The model under review builds one solid part; all positions refer to its coordinate system, in mm. Give positions to 0.01 mm unless a question says otherwise; leave off trailing zeros. Loops run counter-clockwise (first coordinate to the right, second up) from the corner with the lowest first, then second, coordinate; pieces in that order, holes last. Notation, with made-up numbers: M 60.25,-35 L 79.25,-35 A29 cw 79.25,-11 Z; hole C 76,-14.5 d1. An arc over 180 degrees is marked long. Write item = value, one per line. Start each with the question number.
1. We need section A-A on z = 5. Give the boundary of the cut face in (x, y), then the cut area to 3 significant figures.
2. We need section B-B on y = 1.4. Give the boundary of the cut face in (x, z) (3 decimals).
3. Wall thickness on line 1 along Z through (x, y) = (5, 2.8) (3 decimals); line 2 along X through (y, z) = (0.95, -5); line 3 along X through (y, z) = (0.7, -1): over which ranges is each line inside the solid? List them lowest first. Write a range as from..to.
4. We need section C-C on x = 6. Give the boundary of the cut face in (y, z) (3 decimals).
from build123d import *

# Parameters (mm, degrees)
F0_W     = 38.1
F0_H     = 19.05
F0_W_2   = 25.4
F0_H_2   = 1.27
F1_DEPTH = 4.7498
F2_R     = 3.175
F3_R     = 0.7874


with BuildPart() as f1:
    # F0 (on Front) → F1 (new body)
    with BuildSketch(Plane.XZ):
        Rectangle(F0_W, F0_H)
        with Locations((0, -4.7498)):
            Rectangle(F0_W_2, F0_H_2, mode=Mode.SUBTRACT)
        with Locations((0, 4.7498)):
            Rectangle(F0_W_2, F0_H_2, mode=Mode.SUBTRACT)
    extrude(amount=-F1_DEPTH)

    # F2
    f2_edges = [f1.edges().sort_by_distance(p)[0] for p in [
        (19.05, 2.3749, 9.525),
        (19.05, 2.3749, -9.525),
        (-19.05, 2.3749, 9.525),
        (-19.05, 2.3749, -9.525),
    ]]
    fillet(f2_edges, radius=F2_R)

    # F3
    f3_edges = [f1.edges().sort_by_distance(p)[0] for p in [
        (19.05, 0, 0),
        (18.120064, 0, -8.595064),
        (18.120064, 0, 8.595064),
        (0, 0, -9.525),
        (0, 0, 9.525),
        (-18.120064, 0, -8.595064),
        (-18.120064, 0, 8.595064),
        (-19.05, 0, 0),
        (-12.7, 0, -4.7498),
        (0, 0, -4.1148),
        (12.7, 0, -4.7498),
        (0, 0, -5.3848),
        (0, 0, 4.1148),
        (-12.7, 0, 4.7498),
        (0, 0, 5.3848),
        (12.7, 0, 4.7498),
        (19.05, 4.7498, 0),
        (18.120064, 4.7498, -8.595064),
        (18.120064, 4.7498, 8.595064),
        (0, 4.7498, -9.525),
        (0, 4.7498, 9.525),
        (-18.120064, 4.7498, -8.595064),
        (-18.120064, 4.7498, 8.595064),
        (-19.05, 4.7498, 0),
        (-12.7, 4.7498, -4.7498),
        (0, 4.7498, -4.1148),
        (12.7, 4.7498, -4.7498),
        (0, 4.7498, -5.3848),
        (0, 4.7498, 4.1148),
        (-12.7, 4.7498, 4.7498),
        (0, 4.7498, 5.3848),
        (12.7, 4.7498, 4.7498),
    ]]
    fillet(f3_edges, radius=F3_R)


solid = f1.part
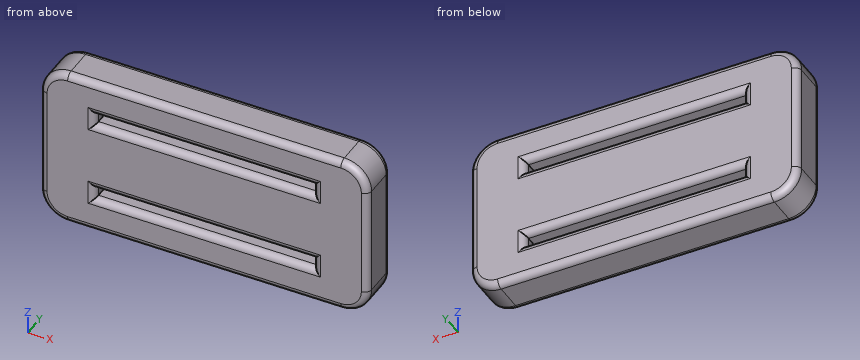
Final values:
q1.outline = M -19.05,0.79 A0.79 ccw -18.26,0 L -13.49,0 A0.79 ccw -12.7,0.79 L -12.7,3.96 A0.79 ccw -13.49,4.75 L -18.26,4.75 A0.79 ccw -19.05,3.96 Z; M 12.7,0.79 A0.79 ccw 13.49,0 L 18.26,0 A0.79 ccw 19.05,0.79 L 19.05,3.96 A0.79 ccw 18.26,4.75 L 13.49,4.75 A0.79 ccw 12.7,3.96 Z
q1.area = 59.3 mm²
q2.outline = M -19.05,-6.35 A3.175 ccw -15.875,-9.525 L 15.875,-9.525 A3.175 ccw 19.05,-6.35 L 19.05,6.35 A3.175 ccw 15.875,9.525 L -15.875,9.525 A3.175 ccw -19.05,6.35 Z; hole M -12.7,-5.385 L 12.7,-5.385 L 12.7,-4.115 L -12.7,-4.115 Z; hole M -12.7,4.115 L 12.7,4.115 L 12.7,5.385 L -12.7,5.385 Z
q3.line_1 = -9.525..-5.385, -4.115..4.115, 5.385..9.525
q3.line_2 = -19.05..-12.7, 12.7..19.05
q3.line_3 = -19.05..19.05
q4.outline = M 0,-8.738 A0.787 ccw 0.787,-9.525 L 3.962,-9.525 A0.787 ccw 4.75,-8.738 L 4.75,-6.172 A0.787 ccw 3.962,-5.385 L 0.787,-5.385 A0.787 ccw 0,-6.172 Z; M 0,-3.327 A0.787 ccw 0.787,-4.115 L 3.962,-4.115 A0.787 ccw 4.75,-3.327 L 4.75,3.327 A0.787 ccw 3.962,4.115 L 0.787,4.115 A0.787 ccw 0,3.327 Z; M 0,6.172 A0.787 ccw 0.787,5.385 L 3.962,5.385 A0.787 ccw 4.75,6.172 L 4.75,8.738 A0.787 ccw 3.962,9.525 L 0.787,9.525 A0.787 ccw 0,8.738 Z
